```python
from build123d import *

# Parameters (mm, degrees)
SKETCH_1_W          = 75
SKETCH_1_H          = 70
SKETCH_1_R          = 4.5
SKETCH_1_R_2        = 2
EXTRUDE_1_DEPTH     = 4
CUT_EXTRUDE_1_DEPTH = 4
SKETCH_3_W          = 8
SKETCH_3_H          = 4
EXTRUDE_2_DEPTH     = 4


with BuildPart() as part:
    # 草图1 → 凸台-拉伸1 (new body)
    with BuildSketch(Plane.XY):
        Rectangle(SKETCH_1_W, SKETCH_1_H)
        Circle(SKETCH_1_R, mode=Mode.SUBTRACT)
        with Locations((19, 0)):
            Circle(SKETCH_1_R_2, mode=Mode.SUBTRACT)
        with Locations((13.435028843, -13.435028843)):
            Circle(SKETCH_1_R_2, mode=Mode.SUBTRACT)
        with Locations((0, -19)):
            Circle(SKETCH_1_R_2, mode=Mode.SUBTRACT)
        with Locations((-13.435028843, -13.435028843)):
            Circle(SKETCH_1_R_2, mode=Mode.SUBTRACT)
        with Locations((-19, 0)):
            Circle(SKETCH_1_R_2, mode=Mode.SUBTRACT)
        with Locations((-13.435028843, 13.435028843)):
            Circle(SKETCH_1_R_2, mode=Mode.SUBTRACT)
        with Locations((0, 19)):
            Circle(SKETCH_1_R_2, mode=Mode.SUBTRACT)
        with Locations((13.435028843, 13.435028843)):
            Circle(SKETCH_1_R_2, mode=Mode.SUBTRACT)
    extrude(amount=EXTRUDE_1_DEPTH)

    # 草图2 → 切除-拉伸1 (cut)
    with BuildSketch(Plane.XY.offset(4)):
        Polygon((-1.5, 35), (1.5, 35), (1.5, 31), (2.8, 31), (2.8, 28.5), (1.5, 28.5), (1.5, 26.5), (-1.5, 26.5), (-1.5, 28.5), (-2.8, 28.5), (-2.8, 31), (-1.5, 31), align=None)
        Polygon((27.5, 35), (27.5, 31), (28.8, 31), (28.8, 28.5), (27.5, 28.5), (27.5, 26.5), (24.5, 26.5), (24.5, 28.5), (23.2, 28.5), (23.2, 31), (24.5, 31), (24.5, 35), align=None)
        Polygon((-27.5, 35), (-24.5, 35), (-24.5, 31), (-23.2, 31), (-23.2, 28.5), (-24.5, 28.5), (-24.5, 26.5), (-27.5, 26.5), (-27.5, 28.5), (-28.8, 28.5), (-28.8, 31), (-27.5, 31), align=None)
        Polygon((-27.5, -35), (-27.5, -31), (-28.8, -31), (-28.8, -28.5), (-27.5, -28.5), (-27.5, -26.5), (-24.5, -26.5), (-24.5, -28.5), (-23.2, -28.5), (-23.2, -31), (-24.5, -31), (-24.5, -35), align=None)
        Polygon((27.5, -35), (24.5, -35), (24.5, -31), (23.2, -31), (23.2, -28.5), (24.5, -28.5), (24.5, -26.5), (27.5, -26.5), (27.5, -28.5), (28.8, -28.5), (28.8, -31), (27.5, -31), align=None)
        Polygon((-1.5, -35), (-1.5, -31), (-2.8, -31), (-2.8, -28.5), (-1.5, -28.5), (-1.5, -26.5), (1.5, -26.5), (1.5, -28.5), (2.8, -28.5), (2.8, -31), (1.5, -31), (1.5, -35), align=None)
    extrude(amount=-CUT_EXTRUDE_1_DEPTH, mode=Mode.SUBTRACT)

    # 草图3 → 凸台-拉伸2 (add)
    with BuildSketch(Plane.XY.offset(4)):
        with Locations((-13, -37)):
            Rectangle(SKETCH_3_W, SKETCH_3_H)
        with Locations((13, -37)):
            Rectangle(SKETCH_3_W, SKETCH_3_H)
        with Locations((13, 37)):
            Rectangle(SKETCH_3_W, SKETCH_3_H)
        with Locations((-13, 37)):
            Rectangle(SKETCH_3_W, SKETCH_3_H)
    extrude(amount=-EXTRUDE_2_DEPTH)


solid = part.part
```
Verification items for the finished model (mm, model axes). A direction names the side the tool comes from. Coordinates: 2 decimals unless noted, no trailing zeros. Write each loop counter-clockwise with the first axis right and the second up, starting at its lowest first coordinate (ties: lowest second). Pieces come first, ordered by that corner, then holes. Notation, with made-up numbers: (23, -21.75) - (78, -21.75) arc R29 cw to (78, 11.25) - close; hole circle Ø11 at (32, -30.75). An arc over 180 degrees is marked (long way). One line per question, with ' | ' between items. Start each with the question number.
1. Gauge pin test, flat ends, axial feed: P1, Ø2, axis at x = -21, z = 1, coming from the -Y side; P2, Ø0.7, axis at x = 24, z = 1.5, coming from the +Y side; P3, Ø1.2, axis at y = 36.5, z = 2, coming from the +X side. Record the tip position at first contact, or that the pin passes through.
2. Draft check along Y on faces 4 (the flat face through (0, -26.5, 2)), 5 (the flat face through (-27.5, 27, 2)), 6 (the flat face through (28.8, -30, 2)). Enter one of: released by +Y, released by -Y, zero draft, split by the parting line, or undercut.
3. Access from +Z, -Z, +X, -X, +Y, -Y to the whole of each face (thin tool, end or side, straight path). Record for faces 1 (the flat face through (17, -37, 2)), 2 (the flat face through (-9, 37, 2)), 3 (the flat face through (-2.8, -30, 2)).
4. Section check C-C (x = 0). Enter the section's corners in (y, z).
5. Section check B-B (x = -19). Enter the section's corners in (y, z).
6. Material ranges on line 1 along X through (y, z) = (30, 3.2); line 2 along X through (y, z) = (-27, 1.85); line 3 along Y through (x, z) = (0, 1.3), recorded low to high.
7. Section check A-A (y = 0). Enter the section's corners in (x, z).
8. Section check D-D (y = -19). Enter the section's corners in (x, z), plus the area to 3 significant figures.
Computed values:
1) P1: y = -35 | P2: y = 35 | P3: x = 17
2) face 4: released by -Y | face 5: zero draft | face 6: undercut
3) face 1: +Z, -Z, +X, -Y | face 2: +Z, -Z, +Y | face 3: +Z, -Z
4) outline: (-26.5, 0) - (-21, 0) - (-21, 4) - (-26.5, 4) - close; (-17, 0) - (-4.5, 0) - (-4.5, 4) - (-17, 4) - close; (4.5, 0) - (17, 0) - (17, 4) - (4.5, 4) - close; (21, 0) - (26.5, 0) - (26.5, 4) - (21, 4) - close
5) outline: (-35, 0) - (-2, 0) - (-2, 4) - (-35, 4) - close; (2, 0) - (35, 0) - (35, 4) - (2, 4) - close
6) line 1: -37.5 to -28.8, -23.2 to -2.8, 2.8 to 23.2, 28.8 to 37.5 | line 2: -37.5 to -27.5, -24.5 to -1.5, 1.5 to 24.5, 27.5 to 37.5 | line 3: -26.5 to -21, -17 to -4.5, 4.5 to 17, 21 to 26.5
7) outline: (-37.5, 0) - (-21, 0) - (-21, 4) - (-37.5, 4) - close; (-17, 0) - (-4.5, 0) - (-4.5, 4) - (-17, 4) - close; (4.5, 0) - (17, 0) - (17, 4) - (4.5, 4) - close; (21, 0) - (37.5, 0) - (37.5, 4) - (21, 4) - close
8) outline: (-37.5, 0) - (-2, 0) - (-2, 4) - (-37.5, 4) - close; (2, 0) - (37.5, 0) - (37.5, 4) - (2, 4) - close | area: 284 mm²
